CAD build for the part. Positions are in the model's coordinates, mm. Give positions to 0.01 mm unless a question says otherwise; leave off trailing zeros. Loops run counter-clockwise (first coordinate to the right, second up) from the corner with the lowest first, then second, coordinate; pieces in that order, holes last. Notation, with made-up numbers: (81.5, -23.5) -> (123.5, -23.5) arc R14 cw to (123.5, -6.5) -> close; hole circle Ø5 at (46.25, 64.25). An arc over 180 degrees is marked (long way). Use one line per item in the form item = value.
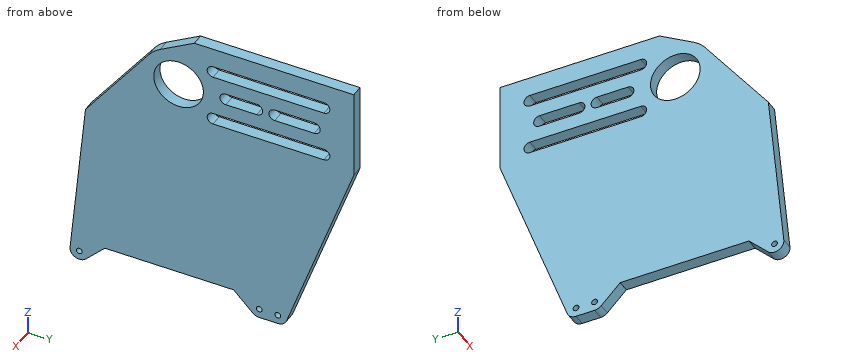
```python
from build123d import *

# Parameters (mm, degrees)
SKETCH4_R           = 1.5
SKETCH4_R_2         = 19.05
SKETCH4_R_3         = 12.7
BOSS_EXTRUDE1_DEPTH = 3


with BuildPart() as part:
    # Sketch4 → Boss-Extrude1 (new, symmetric)
    # profile 1 of 3: a face of its own
    with BuildSketch(Plane(origin=(0, 0, 0), x_dir=(0, 0, -1), z_dir=(1, 0, 0))):
        with BuildLine():
            ThreePointArc((47.817596045, 22.032403955), (48.849976274, 23.577470153), (49.2125, 25.4))
            Line((49.2125, 25.4), (49.2125, 34.925))
            ThreePointArc((49.2125, 34.925), (48.344113354, 37.66676721), (46.055633886, 39.40867551))
            Line((46.055633886, 39.40867551), (-50.063626234, 73.829618952))
            Line((-50.063626234, 73.829618952), (-96.337100071, 73.829618952))
            Line((-96.337100071, 73.829618952), (-96.337100071, -7.774310331))
            Line((-96.337100071, -7.774310331), (-86.423631694, -25.267402912))
            ThreePointArc((-86.423631694, -25.267402912), (-74.706686948, 2.545507373), (-50.8, -15.875))
            ThreePointArc((-50.8, -15.875), (-61.330581006, -32.913837989), (-81.28, -31.115))
            Line((-81.28, -31.115), (-38.1, -63.5))
            Line((-38.1, -63.5), (43.992912904, -71.415514491))
            ThreePointArc((43.992912904, -71.415514491), (48.757334408, -68.706816071), (47.817596045, -63.307403955))
            Line((47.817596045, -63.307403955), (38.1, -53.589807909))
            Line((38.1, -53.589807909), (38.1, 12.314807909))
            Line((38.1, 12.314807909), (47.817596045, 22.032403955))
        make_face()
        with Locations((44.45, -66.675)):
            Circle(SKETCH4_R, mode=Mode.SUBTRACT)
        with BuildLine():
            ThreePointArc((-80.273393759, 1.775), (-83.273393759, -1.225), (-86.273393759, 1.775))
            Line((-86.273393759, 1.775), (-86.273393759, 58.55))
            ThreePointArc((-86.273393759, 58.55), (-83.273393759, 61.55), (-80.273393759, 58.55))
            Line((-80.273393759, 58.55), (-80.273393759, 1.775))
        make_face(mode=Mode.SUBTRACT)
        with BuildLine():
            ThreePointArc((-66.85, 8.3125), (-69.85, 5.3125), (-72.85, 8.3125))
            Line((-72.85, 8.3125), (-72.85, 24.1875))
            Line((-72.85, 24.1875), (-72.85, 33.3625))
            Line((-72.85, 33.3625), (-72.85, 53.6))
            ThreePointArc((-72.85, 53.6), (-69.85, 56.6), (-66.85, 53.6))
            Line((-66.85, 53.6), (-66.85, 33.3625))
            Line((-66.85, 33.3625), (-66.85, 24.1875))
            Line((-66.85, 24.1875), (-66.85, 8.3125))
        make_face(mode=Mode.SUBTRACT)
        with BuildLine():
            ThreePointArc((-53.426606241, 1.775), (-56.426606241, -1.225), (-59.426606241, 1.775))
            Line((-59.426606241, 1.775), (-59.426606241, 58.55))
            ThreePointArc((-59.426606241, 58.55), (-56.426606241, 61.55), (-53.426606241, 58.55))
            Line((-53.426606241, 58.55), (-53.426606241, 1.775))
        make_face(mode=Mode.SUBTRACT)
        with Locations((44.45, 25.4)):
            Circle(SKETCH4_R, mode=Mode.SUBTRACT)
        with Locations((44.45, 34.925)):
            Circle(SKETCH4_R, mode=Mode.SUBTRACT)
    # profile 2 of 3: a face of its own
    with BuildSketch(Plane(origin=(0, 0, 0), x_dir=(0, 0, -1), z_dir=(1, 0, 0))):
        with Locations((-69.85, -15.875)):
            Circle(SKETCH4_R_2)
        with Locations((-69.85, -15.875)):
            Circle(SKETCH4_R_3, mode=Mode.SUBTRACT)
    # profile 3 of 3: a face of its own
    with BuildSketch(Plane(origin=(0, 0, 0), x_dir=(0, 0, -1), z_dir=(1, 0, 0))):
        with BuildLine():
            Line((-72.85, 33.3625), (-72.85, 24.1875))
            ThreePointArc((-72.85, 24.1875), (-69.85, 27.1875), (-66.85, 24.1875))
            Line((-66.85, 24.1875), (-66.85, 33.3625))
            ThreePointArc((-66.85, 33.3625), (-69.85, 30.3625), (-72.85, 33.3625))
        make_face()
    extrude(amount=BOSS_EXTRUDE1_DEPTH, both=True)


solid = part.part
```
1. Drill centre lines: line 1 (Z direction, x = -1.55, y = 3); line 2 (Y direction, x = 0.3, z = -44.45) (1 decimal); line 3 (Z direction, x = 0.45, y = 16). Where is each one in solid material? Low to high.
Result sheet:
line_1 = -38.1 to 53.43, 59.43 to 80.27, 86.27 to 96.34
line_2 = -71.4 to -68.2, -65.2 to -59.9, 18.7 to 23.9, 26.9 to 33.4, 36.4 to 40
line_3 = -41.79 to 53.43, 59.43 to 66.85, 72.85 to 80.27, 86.27 to 96.34
2. Cut at C-C, the plane y = -13. Write the cut outline in (x, z).
Result sheet:
outline = (-3, -38.1) -> (3, -38.1) -> (3, 57.48) -> (-3, 57.48) -> close; (-3, 82.22) -> (3, 82.22) -> (3, 93.38) -> (-3, 93.38) -> close
3. Drop flat-ended pins along their axis: P1, Ø5, axis at y = -53.5, z = 51.5, coming from the +X side; P2, Ø2, axis at x = 1.5, z = 11.5, coming from the +Y side; P3, Ø3, axis at x = 0.5, y = 15.5, coming from the -Z side; P4, Ø1, axis at x = 1.5, z = 32, coming from the -Y side. Give the stop position or say it passes through.
Result sheet:
P1 = 3
P2 = 60.38
P3 = -42.79
P4 = -64.14
4. Cut at D-D, the plane z = 22.5. Write the cut outline in (x, y).
Result sheet:
outline = (-3, -65) -> (3, -65) -> (3, 63.96) -> (-3, 63.96) -> close
5. Cut at B-B, the plane x = -1.8. State how many separate pieces and enclosed holes the cut face has, then the cut area to 3 significant figures.
Result sheet:
separate_pieces = 1
enclosed_holes = 8
area = 14,800 mm^2
6. Cut at A-A, the plane y = 15.5. Write the cut outline in (x, z), then the cut area to 3 significant figures.
Result sheet:
outline = (-3, -41.29) -> (3, -41.29) -> (3, 53.43) -> (-3, 53.43) -> close; (-3, 59.43) -> (3, 59.43) -> (3, 66.85) -> (-3, 66.85) -> close; (-3, 72.85) -> (3, 72.85) -> (3, 80.27) -> (-3, 80.27) -> close; (-3, 86.27) -> (3, 86.27) -> (3, 96.34) -> (-3, 96.34) -> close
area = 718 mm^2
